The model under review builds one solid part; all positions refer to its coordinate system, in mm. Give positions to 0.01 mm unless a question says otherwise; leave off trailing zeros. Loops run counter-clockwise (first coordinate to the right, second up) from the corner with the lowest first, then second, coordinate; pieces in that order, holes last. Notation, with made-up numbers: M 88,1.25 L 104,1.25 A9 cw 104,12.25 Z; hole C 45.25,86.5 d8. An arc over 180 degrees is marked long. Put each result on its own line as item: value. Start each with the question number.
```python
from build123d import *

# Parameters (mm, degrees)
CROQUIS1_R              = 60
SALIENTE_EXTRUIR1_DEPTH = 3.5
CROQUIS2_R              = 2
CORTAR_EXTRUIR1_DEPTH   = 3.5
MATRIZC1_COUNT          = 8
CORTAR_EXTRUIR2_REACH   = 5.5
CROQUIS3_W              = 20.5
CROQUIS3_H              = 40.5
CORTAR_EXTRUIR4_REACH   = 5.5
CROQUIS5_R              = 2


with BuildPart() as part:
    # Croquis1 → Saliente-Extruir1 (new body)
    with BuildSketch(Plane(origin=(0, 0, 0), x_dir=(1, 0, 0), z_dir=(0, 1, 0))):
        Circle(CROQUIS1_R)
    extrude(amount=SALIENTE_EXTRUIR1_DEPTH)

    # Croquis2 → Cortar-Extruir1 (cut)
    with BuildSketch(Plane(origin=(0, 3.5, 0), x_dir=(1, 0, 0), z_dir=(0, 1, 0))):
        with Locations((0, 50)):
            Circle(CROQUIS2_R)
    cortar_extruir1 = extrude(amount=-CORTAR_EXTRUIR1_DEPTH, mode=Mode.SUBTRACT)

    # MatrizC1: Cortar-Extruir1 ×8 about axis
    matrizc1_axis = Axis((0, 0, 0), (0, 1, 0))
    for i in range(1, MATRIZC1_COUNT):
        add(cortar_extruir1.rotate(matrizc1_axis, i * 360 / MATRIZC1_COUNT), mode=Mode.SUBTRACT)

    # Croquis3 → Cortar-Extruir2 (cut, up to next)
    with BuildSketch(Plane(origin=(0, 3.5, 0), x_dir=(1, 0, 0), z_dir=(0, 1, 0)), mode=Mode.PRIVATE) as cortar_extruir2_sk1:
        with Locations((0, 9)):
            Rectangle(CROQUIS3_W, CROQUIS3_H)
    cortar_extruir2_tool1 = extrude(cortar_extruir2_sk1.sketch, amount=-CORTAR_EXTRUIR2_REACH, mode=Mode.PRIVATE) & part.part
    add(cortar_extruir2_tool1.solids().sort_by_distance((0, 3.5, -9))[0], mode=Mode.SUBTRACT)

    # Croquis5 → Cortar-Extruir4 (cut, up to next)
    with BuildSketch(Plane(origin=(0, 3.5, 0), x_dir=(1, 0, 0), z_dir=(0, 1, 0)), mode=Mode.PRIVATE) as cortar_extruir4_sk1:
        with Locations((5, 34.5)):
            Circle(CROQUIS5_R)
    cortar_extruir4_tool1 = extrude(cortar_extruir4_sk1.sketch, amount=-CORTAR_EXTRUIR4_REACH, mode=Mode.PRIVATE) & part.part
    add(cortar_extruir4_tool1.solids().sort_by_distance((5, 3.5, -34.5))[0], mode=Mode.SUBTRACT)
    # Croquis5 → Cortar-Extruir4 (cut, up to next)
    with BuildSketch(Plane(origin=(0, 3.5, 0), x_dir=(1, 0, 0), z_dir=(0, 1, 0)), mode=Mode.PRIVATE) as cortar_extruir4_sk2:
        with Locations((-5, 34.5)):
            Circle(CROQUIS5_R)
    cortar_extruir4_tool2 = extrude(cortar_extruir4_sk2.sketch, amount=-CORTAR_EXTRUIR4_REACH, mode=Mode.PRIVATE) & part.part
    add(cortar_extruir4_tool2.solids().sort_by_distance((-5, 3.5, -34.5))[0], mode=Mode.SUBTRACT)
    # Croquis5 → Cortar-Extruir4 (cut, up to next)
    with BuildSketch(Plane(origin=(0, 3.5, 0), x_dir=(1, 0, 0), z_dir=(0, 1, 0)), mode=Mode.PRIVATE) as cortar_extruir4_sk3:
        with Locations((-5, -16.5)):
            Circle(CROQUIS5_R)
    cortar_extruir4_tool3 = extrude(cortar_extruir4_sk3.sketch, amount=-CORTAR_EXTRUIR4_REACH, mode=Mode.PRIVATE) & part.part
    add(cortar_extruir4_tool3.solids().sort_by_distance((-5, 3.5, 16.5))[0], mode=Mode.SUBTRACT)
    # Croquis5 → Cortar-Extruir4 (cut, up to next)
    with BuildSketch(Plane(origin=(0, 3.5, 0), x_dir=(1, 0, 0), z_dir=(0, 1, 0)), mode=Mode.PRIVATE) as cortar_extruir4_sk4:
        with Locations((5, -16.5)):
            Circle(CROQUIS5_R)
    cortar_extruir4_tool4 = extrude(cortar_extruir4_sk4.sketch, amount=-CORTAR_EXTRUIR4_REACH, mode=Mode.PRIVATE) & part.part
    add(cortar_extruir4_tool4.solids().sort_by_distance((5, 3.5, 16.5))[0], mode=Mode.SUBTRACT)


solid = part.part
```
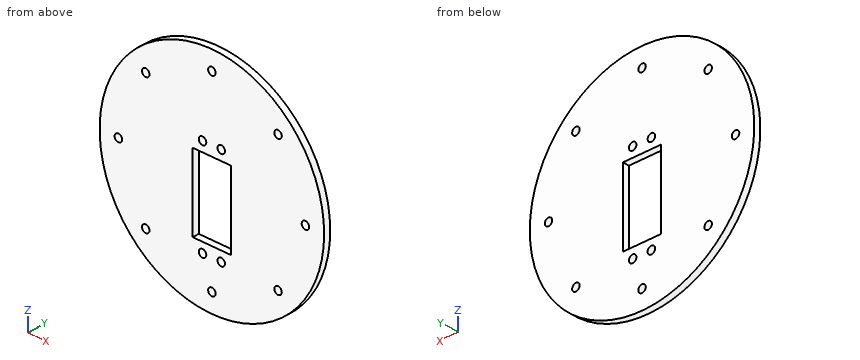
Item 1: Clearance check with flat-ended pins moving along their axes: pin 1 Ø1.8 at (y, z) = (1.5, -6) entering from +X; pin 2 Ø2 at (x, y) = (-16, 2.5) entering from +Z; pin 3 Ø1.8 at (y, z) = (1, -5.5) entering from -X. State where each tip first meets the part, or that it passes through.
Item 2: Consider section C-C, the plane z = 50. Write out the cut boundary in (x, y).
Item 3: Consider section B-B, the plane z = 0. Write out the cut boundary in (x, y).
Item 4: Consider section D-D, the plane y = 1.15. Give the number of separate pieces and of enclosed holes in the cut face, plus the area to 3 significant figures.
Item 5: To check wall thickness, follow L1, parallel to X at y = 2.4, z = 0; L2, parallel to Z at x = 0, y = 2.25; L3, parallel to Z at x = -5, y = 1.35. State the ranges of each line that lie inside material, in increasing order. Write a range as [from, to].
Item 6: Consider section A-A, the plane x = 0. Write out the cut boundary in (y, z).
Report:
1. pin 1: x = 59.78
1. pin 2: z = 58.09
1. pin 3: x = -59.82
2. outline: M -33.17,0 L -2,0 L -2,3.5 L -33.17,3.5 Z; M 2,0 L 33.17,0 L 33.17,3.5 L 2,3.5 Z
3. outline: M -60,0 L -52,0 L -52,3.5 L -60,3.5 Z; M -48,0 L -10.25,0 L -10.25,3.5 L -48,3.5 Z; M 10.25,0 L 48,0 L 48,3.5 L 10.25,3.5 Z; M 52,0 L 60,0 L 60,3.5 L 52,3.5 Z
4. separate pieces: 1
4. enclosed holes: 13
4. area: 10,300 mm²
5. L1: [-60, -52], [-48, -10.25], [10.25, 48], [52, 60]
5. L2: [-60, -52], [-48, -29.25], [11.25, 48], [52, 60]
5. L3: [-59.79, -36.5], [-32.5, -29.25], [11.25, 14.5], [18.5, 59.79]
6. outline: M 0,-60 L 3.5,-60 L 3.5,-52 L 0,-52 Z; M 0,-48 L 3.5,-48 L 3.5,-29.25 L 0,-29.25 Z; M 0,11.25 L 3.5,11.25 L 3.5,48 L 0,48 Z; M 0,52 L 3.5,52 L 3.5,60 L 0,60 Z
